Geometry check sheet. Reference: the model listing, model coordinates, mm. Face numbers are marked on the shaded views. A direction names the side the tool comes from. Coordinates: 2 decimals unless noted, no trailing zeros. Write each loop counter-clockwise with the first axis right and the second up, starting at its lowest first coordinate (ties: lowest second). Pieces come first, ordered by that corner, then holes. Notation, with made-up numbers: (75.5, 47) -> (127.5, 47) arc R33 ccw to (127.5, 83) -> close; hole circle Ø9 at (-38, 8.5). An arc over 180 degrees is marked (long way). Answer in a Markdown table with one row per item. Add a question column.
Q1. Thickness scan on line 1 (X direction, y = 27, z = 11); line 2 (X direction, y = 19, z = 7); line 3 (Y direction, x = -16, z = 18.5). Record the ranges inside material, lowest first.
Q2. Section check A-A, the plane y = 21.5. Record the boundary of the cut face in (x, z).
Q3. Section check D-D, the plane y = 7. Record the boundary of the cut face in (x, z) (3 decimals), and give its area (3 significant figures).
Q4. Gauge pin test, flat ends, axial feed: P1, Ø6, axis at x = 17.5, y = -4, coming from the -Z side; P2, Ø4, axis at y = 19.5, z = 16.5, coming from the -X side; P3, Ø2, axis at y = -1, z = 15.5, coming from the -X side. Record the tip position at first contact, or that the pin passes through.
Q5. Section check B-B, the plane z = 4.25. Record the boundary of the cut face in (x, y), and give its area (3 significant figures).
Q6. Section check C-C, the plane x = 19. Record the boundary of the cut face in (y, z), and give its area (3 significant figures).
Q7. Release check for a two-part mould opening along Y. For the marked faces 3, 4 and 5 record: pulls with the +Y half, pulls with the -Y half, needs draft (parallel to the pull), parting line crosses it, or undercut.
Q8. Tool access check on the marked faces 1 and 2. Record the directions out of +Z, -Z, +X, -X, +Y, -Y that give a thin tool (end or side, any length) a straight path to the whole face; none if there is none.
```python
from build123d import *

# Parameters (mm, degrees)
F1_DEPTH = 20


with BuildPart() as f1:
    # F0 (on Top) → F1 (new body)
    with BuildSketch(Plane.XY):
        with BuildLine():
            ThreePointArc((-17.320508, -30), (0, -20), (17.320508, -30))
            Line((17.320508, -30), (30, -30))
            Line((30, -30), (30, 30))
            Line((30, 30), (20, 30))
            Line((20, 30), (0, 0))
            Line((0, 0), (-20, 30))
            Line((-20, 30), (-30, 30))
            Line((-30, 30), (-44.90712, 13.333333))
            ThreePointArc((-44.90712, 13.333333), (-50, 0), (-44.90712, -13.333333))
            Line((-44.90712, -13.333333), (-30, -30))
            Line((-30, -30), (-17.320508, -30))
        make_face()
    extrude(amount=F1_DEPTH)


solid = f1.part
```
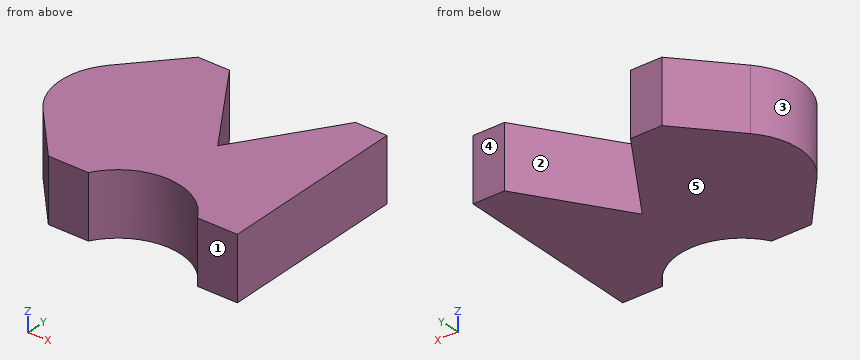
Calculated:
| question | item | result |
|---|---|---|
| 1 | line 1 | x = -32.68 to -18, 18 to 30 |
| 1 | line 2 | x = -39.84 to -12.67, 12.67 to 30 |
| 1 | line 3 | y = -28 to 24 |
| 2 | outline | (-37.6, 0) -> (-14.33, 0) -> (-14.33, 20) -> (-37.6, 20) -> close; (14.33, 0) -> (30, 0) -> (30, 20) -> (14.33, 20) -> close |
| 3 | outline | (-48.735, 0) -> (-4.667, 0) -> (-4.667, 20) -> (-48.735, 20) -> close; (4.667, 0) -> (30, 0) -> (30, 20) -> (4.667, 20) -> close |
| 3 | area | 1,390 mm² |
| 4 | P1 | stops at z = 0 |
| 4 | P2 | stops at x = -41.18 |
| 4 | P3 | stops at x = -50 |
| 5 | outline | (-44.91, -13.33) -> (-30, -30) -> (-17.32, -30) arc R20 cw to (17.32, -30) -> (30, -30) -> (30, 30) -> (20, 30) -> (0, 0) -> (-20, 30) -> (-30, 30) -> (-44.91, 13.33) arc R20 ccw to start |
| 5 | area | 3,490 mm² |
| 6 | outline | (-30, 0) -> (28.5, 0) -> (28.5, 20) -> (-30, 20) -> close |
| 6 | area | 1,170 mm² |
| 7 | face 3 | parting line crosses it |
| 7 | face 4 | pulls with the +Y half |
| 7 | face 5 | needs draft |
| 8 | face 1 | +Z, -Z, +X, -X, -Y |
| 8 | face 2 | +Z, -Z, +Y |
